The model under review builds one solid part; all positions refer to its coordinate system, in mm. A direction names the side the tool comes from. Give positions to 0.01 mm unless a question says otherwise; leave off trailing zeros. Order: outer loops, then holes, each group sorted by start corner. A loop starts at its lowest first (then second) coordinate and runs counter-clockwise, first axis right, second up. Notation, with made-up numbers: (-21, 45) - (10, 45) arc R29 ccw to (10, 76) - close; hole circle Ø5 at (36, 72). An arc over 180 degrees is marked (long way). Write item = value, one per line. Start each with the question number.
1. Machinability: for faces 1 (the conical face through (-18.27, -8.66, -0.07)), 2 (the flat face through (0.21, -12.218, 5.125)), which of the approach directions +Z, -Z, +X, -X, +Y, -Y give a long, thin tool a straight path to every point of the face, cutting with its end or side? Answer none if there is none.
2. We need section B-B, the plane y = 4. Give the boundary of the cut face in (x, z).
3. Wall thickness on probe 1 along Z at (x, y) = (-14, 59); probe 2 along Z at (x, y) = (17, -2.5); probe 3 along X at (y, z) = (48, 4.75): over which ranges is each line inside the solid? List them lowest first.
4. Mouldability with a two-part tool opening along Z and no side actions: class faces 3 (the flat face through (-0.21, -8.92, -3.22)), 4 (the flat face through (2, 91, -9)), 5 (the flat face through (0, 58, 11.154)) as pulls with the +Z half, pulls with the -Z half, needs draft (parallel to the pull), parting line crosses it, or undercut.
5. For P1, Ø10, axis at y = 0.5, z = -1.5, coming from the +X side; P2, Ø0.9, axis at x = 14.5, z = 0, coming from the +Y side; P3, Ø6, axis at x = 0, y = -6.5, coming from the -Z side, all flat-tipped, find the tip position at first contact; note any pin that passes through.
6. We need section A-A, the plane y = 66. Give the boundary of the cut face in (x, z).
from build123d import *

# Parameters (mm, degrees)
BOSS_EXTRUDE1_DEPTH           = 18
BOSS_EXTRUDE1_TAPER           = 11
BOSS_EXTRUDE1_OTHER_WAY_DEPTH = 26
BOSS_EXTRUDE1_OTHER_WAY_TAPER = -8
SHELL1_START                  = -15
SHELL1_DEPTH                  = 30
SKETCH2_W                     = 25
SKETCH2_H                     = 3.2
BOSS_EXTRUDE2_DEPTH           = 20
BOSS_EXTRUDE2_TAPER           = 11
BOSS_EXTRUDE3_DEPTH           = 65


with BuildPart() as part:
    # Sketch1 → Boss-Extrude1 (new body)
    with BuildSketch(Plane(origin=(0, 0, 0), x_dir=(1, 0, 0), z_dir=(0, 1, 0))):
        with BuildLine():
            ThreePointArc((-15, 7.5), (-22.5, 0), (-15, -7.5))
            Line((-15, -7.5), (15, -7.5))
            ThreePointArc((15, -7.5), (22.5, 0), (15, 7.5))
            Line((15, 7.5), (-15, 7.5))
        make_face()
    extrude(amount=-BOSS_EXTRUDE1_DEPTH, taper=BOSS_EXTRUDE1_TAPER)

    # Sketch1 → Boss-Extrude1 other way (add)
    with BuildSketch(Plane(origin=(0, 0, 0), x_dir=(1, 0, 0), z_dir=(0, 1, 0))):
        with BuildLine():
            ThreePointArc((-15, 7.5), (-22.5, 0), (-15, -7.5))
            Line((-15, -7.5), (15, -7.5))
            ThreePointArc((15, -7.5), (22.5, 0), (15, 7.5))
            Line((15, 7.5), (-15, 7.5))
        make_face()
    extrude(amount=BOSS_EXTRUDE1_OTHER_WAY_DEPTH, taper=BOSS_EXTRUDE1_OTHER_WAY_TAPER)

    # Shell1: read off the stored shape, not the designer's step
    # Shell1 outline → Shell1 (cut)
    with BuildSketch(Plane.YZ.offset(SHELL1_START)):
        Polygon((26, -8.629492771), (26, 8.629492771), (0.412760457, 5.033440768), (-18, 1.454362698), (-18, -1.454362698), (0.412760457, -5.033440768), align=None)
    extrude(amount=SHELL1_DEPTH, mode=Mode.SUBTRACT)

    # Shell1 2 outline → Shell1 2 (revolve, cut)
    with BuildSketch(Plane(origin=(-15, 0, 0), x_dir=(1, 0, 0), z_dir=(0, 0, 1))):
        Polygon((1.454362698, -18), (5.033440768, 0.412760457), (8.629492771, 26), (0, 26), (0, -18), align=None)
    revolve(axis=Axis((-15, 0, 0), (0, 1, 0)), mode=Mode.SUBTRACT)

    # Shell1 3 outline → Shell1 3 (revolve, cut)
    with BuildSketch(Plane(origin=(15, 0, 0), x_dir=(1, 0, 0), z_dir=(0, 0, 1))):
        Polygon((1.454362698, -18), (5.033440768, 0.412760457), (8.629492771, 26), (0, 26), (0, -18), align=None)
    revolve(axis=Axis((15, 0, 0), (0, 1, 0)), mode=Mode.SUBTRACT)

    # Sketch2 → Boss-Extrude2 (add)
    with BuildSketch(Plane.XZ.offset(18)):
        with BuildLine():
            ThreePointArc((-15, 4.001154436), (-19.001154436, 0), (-15, -4.001154436))
            Line((-15, -4.001154436), (15, -4.001154436))
            ThreePointArc((15, -4.001154436), (19.001154436, 0), (15, 4.001154436))
            Line((15, 4.001154436), (-15, 4.001154436))
        make_face()
        Rectangle(SKETCH2_W, SKETCH2_H, mode=Mode.SUBTRACT)
    extrude(amount=BOSS_EXTRUDE2_DEPTH, taper=BOSS_EXTRUDE2_TAPER)

    # Sketch3 → Boss-Extrude3 (add)
    with BuildSketch(Plane(origin=(0, 26, 0), x_dir=(1, 0, 0), z_dir=(0, 1, 0))):
        with BuildLine():
            Line((-15, -11.154061702), (15, -11.154061702))
            ThreePointArc((15, -11.154061702), (26.154061702, 0), (15, 11.154061702))
            Line((15, 11.154061702), (-15, 11.154061702))
            ThreePointArc((-15, 11.154061702), (-26.154061702, 0), (-15, -11.154061702))
        make_face()
        with BuildLine():
            Line((-15, -8.629492771), (15, -8.629492771))
            ThreePointArc((15, -8.629492771), (23.629492771, 0), (15, 8.629492771))
            Line((15, 8.629492771), (-15, 8.629492771))
            ThreePointArc((-15, 8.629492771), (-23.629492771, 0), (-15, -8.629492771))
        make_face(mode=Mode.SUBTRACT)
    extrude(amount=BOSS_EXTRUDE3_DEPTH)


solid = part.part
Model answer:
q1.face_1 = +Y
q1.face_2 = +Z, +X, -X, -Y
q2.outline = (-15, -8.06) - (15, -8.06) arc R8.06 ccw to (15, 8.06) - (-15, 8.06) arc R8.06 ccw to start; hole (-15, -5.54) - (15, -5.54) arc R5.54 ccw to (15, 5.54) - (-15, 5.54) arc R5.54 ccw to start
q3.probe_1 = -11.15 to -8.63, 8.63 to 11.15
q3.probe_2 = -6.72 to -3.99, 3.99 to 6.72
q3.probe_3 = -25.09 to -22.2, 22.2 to 25.09
q4.face_3 = undercut
q4.face_4 = needs draft
q4.face_5 = pulls with the +Z half
q5.P1 = 23.25
q5.P2 = -18
q5.P3 = -6.82
q6.outline = (-15, -11.15) - (15, -11.15) arc R11.15 ccw to (15, 11.15) - (-15, 11.15) arc R11.15 ccw to start; hole (-15, -8.63) - (15, -8.63) arc R8.63 ccw to (15, 8.63) - (-15, 8.63) arc R8.63 ccw to start
